The model under review builds one solid part; all positions refer to its coordinate system, in mm. A direction names the side the tool comes from. Coordinates: 2 decimals unless noted, no trailing zeros. Write each loop counter-clockwise with the first axis right and the second up, starting at its lowest first coordinate (ties: lowest second). Pieces come first, ordered by that corner, then holes. Notation, with made-up numbers: M 68,56 L 85,56 A27 cw 85,74 Z; hole C 36.25,-18 d7. An arc over 180 degrees is marked long. Answer as CSV lines item,"result". Start each with the question number.
from build123d import *

# Parameters (mm, degrees)
SKETCH1_W           = 23
SKETCH1_H           = 27.4
SKETCH1_W_2         = 4.5
SKETCH1_H_2         = 1.5
BOSS_EXTRUDE1_DEPTH = 6
CHAMFER1_SIZE       = 0.5
SKETCH3_R           = 1.25
CUT_EXTRUDE1_DEPTH  = 28.4
BOSS_EXTRUDE2_START = -7
SKETCH3_3_R         = 4.5
BOSS_EXTRUDE2_DEPTH = 8
CHAMFER2_SIZE       = 0.5
BOSS_EXTRUDE3_START = 1
SKETCH3_4_R         = 2.45
BOSS_EXTRUDE3_DEPTH = 3.2


with BuildPart() as part:
    # Sketch1 → Boss-Extrude1 (new body, symmetric)
    with BuildSketch(Plane(origin=(0, 0, 0), x_dir=(0, 0, -1), z_dir=(1, 0, 0))):
        with Locations((-11.5, 13.7)):
            Rectangle(SKETCH1_W, SKETCH1_H)
        with Locations((-25.25, 21.15)):
            Rectangle(SKETCH1_W_2, SKETCH1_H_2)
        with Locations((2.25, 21.15)):
            Rectangle(SKETCH1_W_2, SKETCH1_H_2)
    extrude(amount=BOSS_EXTRUDE1_DEPTH, both=True)

    # Chamfer1
    chamfer1_edges = [part.edges().sort_by_distance(p)[0] for p in [
        (-6, 24.65, 23),
        (-6, 27.4, 11.5),
        (-6, 24.65, 0),
        (-6, 10.2, 0),
        (-6, 0, 11.5),
        (-6, 10.2, 23),
        (6, 10.2, 23),
        (0, 27.4, 23),
        (0, 27.4, 0),
        (0, 0, 0),
        (0, 0, 23),
        (6, 0, 11.5),
        (6, 10.2, 0),
        (6, 24.65, 0),
        (6, 27.4, 11.5),
        (6, 24.65, 23),
    ]]
    chamfer(chamfer1_edges, length=CHAMFER1_SIZE)

    # Sketch3 → Cut-Extrude1 (cut, through all)
    with BuildSketch(Plane(origin=(0, 27.4, 0), x_dir=(1, 0, 0), z_dir=(0, 1, 0))):
        with Locations((-3.5, -25.5)):
            Circle(SKETCH3_R)
        with Locations((3.5, -25.5)):
            Circle(SKETCH3_R)
        with Locations((3.5, 2.5)):
            Circle(SKETCH3_R)
        with Locations((-3.5, 2.5)):
            Circle(SKETCH3_R)
    extrude(amount=-CUT_EXTRUDE1_DEPTH, mode=Mode.SUBTRACT)

    # Sketch3<3> → Boss-Extrude2 (add)
    with BuildSketch(Plane(origin=(0, 27.4, 0), x_dir=(1, 0, 0), z_dir=(0, 1, 0)).offset(BOSS_EXTRUDE2_START)):
        with Locations((0, -5.5)):
            Circle(SKETCH3_3_R)
    extrude(amount=BOSS_EXTRUDE2_DEPTH)

    # Chamfer2
    chamfer2_edges = [part.edges().sort_by_distance(p)[0] for p in [
        (-4.5, 28.4, 5.5),
    ]]
    chamfer(chamfer2_edges, length=CHAMFER2_SIZE)

    # Sketch3<4> → Boss-Extrude3 (add)
    with BuildSketch(Plane(origin=(0, 27.4, 0), x_dir=(1, 0, 0), z_dir=(0, 1, 0)).offset(BOSS_EXTRUDE3_START)):
        with Locations((0, -5.5)):
            Circle(SKETCH3_4_R)
    extrude(amount=BOSS_EXTRUDE3_DEPTH)


solid = part.part
1) Tool access review of faces 1 (the flat face through (0, 21, -4.5)), 2 (the flat face through (0, 24, 0)), 3 (the flat face through (0, 10, 0)), 4 (the cylindrical face through (2.08, 27.65, 9.49)), 5 (the flat face through (0, 0, 12)): name each direction out of +Z, -Z, +X, -X, +Y, -Y from which nothing blocks a thin tool from reaching the whole face with its end or side.
2) Take a section at D-D on x = 0. Give the boundary of the cut face in (y, z), and give its area (3 significant figures).
3) Take a section at A-A on z = 25.5. Give the boundary of the cut face in (x, y), and give its area (3 significant figures).
4) Take a section at B-B on y = 7.5. Give the boundary of the cut face in (x, z), and give its area (4 significant figures).
5) Mouldability with a two-part tool opening along X and no side actions: class faces 6 (the flat face through (0, 24, 23)), 7 (the cylindrical face through (-0.32, 29.98, 3.07)), 8 (the cylindrical face through (4.69, 21.16, -2.88)) as +X half, -X half, draft (parallel to the pull), parting line (faces both ways), or undercut.
6) To check wall thickness, follow line 1 (Z direction, x = -3.5, y = 20.9); line 2 (X direction, y = 21.05, z = 25.5); line 3 (Y direction, x = 5.5, z = 20.5). State the ranges of each line that lie inside material, in increasing order. Write a range as [from, to].
7) Take a section at C-C on z = 5.5. Give the boundary of the cut face in (x, y).
8) Clearance check with flat-ended pins moving along their axes: pin 1 Ø2.5 at (x, y) = (0.5, 25) entering from -Z; pin 2 Ø1.5 at (x, z) = (-2.5, 25) entering from +Y; pin 3 Ø2 at (x, z) = (3.5, -2.5) entering from -Y; pin 4 Ø3 at (x, z) = (-3.5, 25.5) entering from -Y. State where each tip first meets the part, or that it passes through.
Results:
1,face 1,"-Z, +X, -X, +Y, -Y"
1,face 2,"-Z, +X, -X, +Y"
1,face 3,"-Z, +X, -X, -Y"
1,face 4,"+Y"
1,face 5,"+Z, -Z, +X, -X, -Y"
2,outline,"M 0,0.5 L 0.5,0 L 20.4,0 L 20.4,-4.5 L 21.9,-4.5 L 21.9,0 L 26.9,0 L 27.4,0.5 L 27.4,1 L 27.9,1 L 28.4,1.5 L 28.4,3.05 L 31.6,3.05 L 31.6,7.95 L 28.4,7.95 L 28.4,9.5 L 27.9,10 L 27.4,10 L 27.4,22.5 L 26.9,23 L 21.9,23 L 21.9,27.5 L 20.4,27.5 L 20.4,23 L 0.5,23 L 0,22.5 Z"
2,area,"668 mm²"
3,outline,"M -6,20.4 L -4.75,20.4 L -4.75,21.9 L -6,21.9 Z; M -2.25,20.4 L 2.25,20.4 L 2.25,21.9 L -2.25,21.9 Z; M 4.75,20.4 L 6,20.4 L 6,21.9 L 4.75,21.9 Z"
3,area,"10.5 mm²"
4,outline,"M -6,0.5 L -5.5,0 L 5.5,0 L 6,0.5 L 6,22.5 L 5.5,23 L -5.5,23 L -6,22.5 Z"
4,area,"275.5 mm²"
5,face 6,"draft"
5,face 7,"parting line"
5,face 8,"undercut"
6,line 1,"z = [-4.5, -3.75], [-1.25, 24.25], [26.75, 27.5]"
6,line 2,"x = [-6, -4.75], [-2.25, 2.25], [4.75, 6]"
6,line 3,"y = [0, 27.4]"
7,outline,"M -6,0.5 L -5.5,0 L 5.5,0 L 6,0.5 L 6,26.9 L 5.5,27.4 L 4.5,27.4 L 4.5,27.9 L 4,28.4 L 2.45,28.4 L 2.45,31.6 L -2.45,31.6 L -2.45,28.4 L -4,28.4 L -4.5,27.9 L -4.5,27.4 L -5.5,27.4 L -6,26.9 Z"
8,pin 1,"stops at z = 0"
8,pin 2,"stops at y = 21.9"
8,pin 3,"passes through"
8,pin 4,"stops at y = 20.4"
